Could you check a few things on this model? Use its own coordinates, in mm. Give positions to 0.01 mm unless a question says otherwise; leave off trailing zeros. Loops run counter-clockwise (first coordinate to the right, second up) from the corner with the lowest first, then second, coordinate; pieces in that order, holes last. Notation, with made-up numbers: M -4,71 L 49,71 A35 cw 49,104 Z; hole C 75,68 d9. An arc over 180 degrees is marked long. Answer in a Markdown table with one row per item. Add a question column.
1. If we section it at B-B on x = -17.5: List the corners of the cut face in (y, z) for me, then the cut area to 3 significant figures.
2. If we section it at D-D on y = 4: Count the separate pieces of the cut face and the enclosed holes in it, then the cut area to 3 significant figures.
3. I'm going to push flat-ended pins straight in: pin 1 Ø5 at (x, z) = (24.89, 60.6) entering from +Y; pin 2 Ø1.6 at (x, y) = (24, 3.5) entering from +Z; pin 3 Ø2.5 at (x, y) = (26, 3.5) entering from -Z. Where does each tip first touch, or does it pass through?
4. If we section it at A-A on z = 71: List the corners of the cut face in (x, y) for me.
5. If we section it at C-C on z = 9.22: List the corners of the cut face in (x, y) for me, then the cut area to 3 significant figures.
6. I need wall thicknesses on line 1 along X through (y, z) = (0.65, 83); line 2 along Z through (x, y) = (26, 2.75); line 3 along Z through (x, y) = (-25.5, 1.75). Which ranges of each line are inside material? Lowest first, please. Write a range as from..to.
```python
from build123d import *

# Parameters (mm, degrees)
SKETCH1_R           = 1.5
SKETCH1_R_2         = 6.5
SKETCH1_R_3         = 5.5
BOSS_EXTRUDE1_DEPTH = 6
FILLET1_R           = 10
SKETCH2_R           = 4
CUT_EXTRUDE1_DEPTH  = 3
SKETCH1_3_R         = 5.5
SKETCH1_3_R_2       = 3.5
BOSS_EXTRUDE2_DEPTH = 3
SKETCH3_W           = 3.3
SKETCH3_H           = 7.5
SKETCH3_H_2         = 1
SKETCH3_W_2         = 1.15
SKETCH3_H_3         = 4.1
SKETCH3_H_4         = 2.4
CUT_EXTRUDE2_DEPTH  = 10


with BuildPart() as part:
    # Sketch1 → Boss-Extrude1 (new body)
    with BuildSketch(Plane(origin=(0, 0, 0), x_dir=(1, 0, 0), z_dir=(0, 1, 0))):
        Polygon((17.441626812, 0.78), (-17.441626812, 0.78), (-35, -35.22), (-35, -94.22), (-12.5, -94.22), (-12.5, -88.22), (12.5, -88.22), (12.5, -94.22), (35, -94.22), (35, -35.22), align=None)
        with Locations(Location((-24.889613301, -70.60075616, 0), (0, 0, 270))):
            Circle(SKETCH1_R, mode=Mode.SUBTRACT)
        with Locations(Location((-24.889613301, -60.60075616, 0), (0, 0, 270))):
            Circle(SKETCH1_R, mode=Mode.SUBTRACT)
        with Locations(Location((24.889613301, -70.60075616, 0), (0, 0, 270))):
            Circle(SKETCH1_R, mode=Mode.SUBTRACT)
        with Locations(Location((10.3, -65.60075616, 0), (0, 0, 270))):
            Circle(SKETCH1_R_2, mode=Mode.SUBTRACT)
        with Locations(Location((24.889613301, -60.60075616, 0), (0, 0, 270))):
            Circle(SKETCH1_R, mode=Mode.SUBTRACT)
        with Locations(Location((-17.5, -33.65200814, 0), (0, 0, 270))):
            Circle(SKETCH1_R_3, mode=Mode.SUBTRACT)
        with Locations(Location((-8.607476274, -9.22, 0), (0, 0, 270))):
            Circle(SKETCH1_R_3, mode=Mode.SUBTRACT)
        with Locations(Location((17.5, -33.65200814, 0), (0, 0, 270))):
            Circle(SKETCH1_R_3, mode=Mode.SUBTRACT)
        with Locations(Location((8.607476274, -9.22, 0), (0, 0, 270))):
            Circle(SKETCH1_R_3, mode=Mode.SUBTRACT)
    extrude(amount=BOSS_EXTRUDE1_DEPTH)

    # Fillet1
    fillet1_edges = [part.edges().sort_by_distance(p)[0] for p in [
        (-35, 3, 35.22),
        (-17.441626812, 3, -0.78),
        (17.441626812, 3, -0.78),
        (35, 3, 35.22),
    ]]
    fillet(fillet1_edges, radius=FILLET1_R)

    # Sketch2 → Cut-Extrude1 (cut)
    with BuildSketch(Plane(origin=(0, 6, 0), x_dir=(1, 0, 0), z_dir=(0, 1, 0))):
        with Locations(Location((24.889613301, -60.60075616, 0), (0, 0, 270))):
            Circle(SKETCH2_R)
        with Locations(Location((24.889613301, -70.60075616, 0), (0, 0, 270))):
            Circle(SKETCH2_R)
        with Locations(Location((-24.889613301, -60.60075616, 0), (0, 0, 270))):
            Circle(SKETCH2_R)
        with Locations(Location((-24.889613301, -70.60075616, 0), (0, 0, 270))):
            Circle(SKETCH2_R)
    extrude(amount=-CUT_EXTRUDE1_DEPTH, mode=Mode.SUBTRACT)

    # Sketch1_3 → Boss-Extrude2 (add)
    # profile 1 of 4: a face of its own
    with BuildSketch(Plane(origin=(0, 0, 0), x_dir=(1, 0, 0), z_dir=(0, 1, 0))):
        with Locations(Location((-17.5, -33.65200814, 0), (0, 0, 270))):
            Circle(SKETCH1_3_R)
        with Locations(Location((-17.5, -33.65200814, 0), (0, 0, 270))):
            Circle(SKETCH1_3_R_2, mode=Mode.SUBTRACT)
    # profile 2 of 4: a face of its own
    with BuildSketch(Plane(origin=(0, 0, 0), x_dir=(1, 0, 0), z_dir=(0, 1, 0))):
        with Locations(Location((-8.607476274, -9.22, 0), (0, 0, 270))):
            Circle(SKETCH1_3_R)
        with Locations(Location((-8.607476274, -9.22, 0), (0, 0, 270))):
            Circle(SKETCH1_3_R_2, mode=Mode.SUBTRACT)
    # profile 3 of 4: a face of its own
    with BuildSketch(Plane(origin=(0, 0, 0), x_dir=(1, 0, 0), z_dir=(0, 1, 0))):
        with Locations(Location((17.5, -33.65200814, 0), (0, 0, 270))):
            Circle(SKETCH1_3_R)
        with Locations(Location((17.5, -33.65200814, 0), (0, 0, 270))):
            Circle(SKETCH1_3_R_2, mode=Mode.SUBTRACT)
    # profile 4 of 4: a face of its own
    with BuildSketch(Plane(origin=(0, 0, 0), x_dir=(1, 0, 0), z_dir=(0, 1, 0))):
        with Locations(Location((8.607476274, -9.22, 0), (0, 0, 270))):
            Circle(SKETCH1_3_R)
        with Locations(Location((8.607476274, -9.22, 0), (0, 0, 270))):
            Circle(SKETCH1_3_R_2, mode=Mode.SUBTRACT)
    extrude(amount=BOSS_EXTRUDE2_DEPTH)

    # Sketch3 → Cut-Extrude2 (cut)
    with BuildSketch(Plane(origin=(0, 6, 0), x_dir=(1, 0, 0), z_dir=(0, 1, 0))):
        with Locations((23.75, -90.47)):
            Rectangle(SKETCH3_W, SKETCH3_H)
        Polygon((26.55, -85.72), (25.4, -85.72), (25.4, -86.72), (27.75, -86.72), (27.75, -85.72), align=None)
        with Locations((23.75, -86.22)):
            Rectangle(SKETCH3_W, SKETCH3_H_2)
        Polygon((22.1, -85.72), (20.95, -85.72), (19.75, -85.72), (19.75, -86.72), (22.1, -86.72), align=None)
        with Locations((21.525, -83.67)):
            Rectangle(SKETCH3_W_2, SKETCH3_H_3)
        with Locations((23.75, -83.67)):
            Rectangle(SKETCH3_W, SKETCH3_H_3)
        with Locations((25.975, -83.67)):
            Rectangle(SKETCH3_W_2, SKETCH3_H_3)
        with Locations((23.75, -80.42)):
            Rectangle(SKETCH3_W, SKETCH3_H_4)
    cut_extrude2 = extrude(amount=-CUT_EXTRUDE2_DEPTH, mode=Mode.SUBTRACT)

    # Mirror1: Cut-Extrude2 across plane
    add(cut_extrude2.mirror(Plane(origin=(0, 0, 0), x_dir=(0, 0, 1), z_dir=(1, 0, 0))), mode=Mode.SUBTRACT)


solid = part.part
```
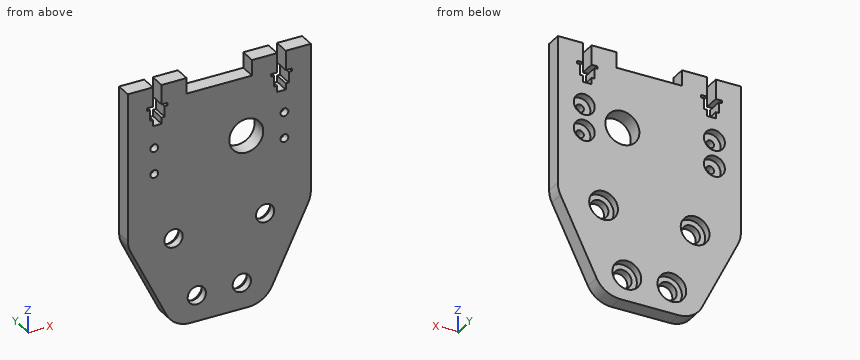
Results:
| question | item | result |
|---|---|---|
| 1 | outline | M 0,1.46 L 6,1.46 L 6,28.15 L 3,28.15 L 3,30.15 L 0,30.15 Z; M 0,37.15 L 3,37.15 L 3,39.15 L 6,39.15 L 6,94.22 L 0,94.22 Z |
| 1 | area | 503 mm2 |
| 2 | separate pieces | 1 |
| 2 | enclosed holes | 9 |
| 2 | area | 5,010 mm2 |
| 3 | pin 1 | y = 3 |
| 3 | pin 2 | z = 79.22 |
| 3 | pin 3 | z = 14.2 |
| 4 | outline | M -35,0 L -26.34,0 L -26.34,3 L -28.87,3 L -28.87,6 L -35,6 Z; M -23.44,0 L 6.68,0 L 6.68,6 L -20.91,6 L -20.91,3 L -23.44,3 Z; M 13.92,0 L 23.44,0 L 23.44,3 L 20.91,3 L 20.91,6 L 13.92,6 Z; M 26.34,0 L 35,0 L 35,6 L 28.87,6 L 28.87,3 L 26.34,3 Z |
| 5 | outline | M -22.32,0 L -12.11,0 L -12.11,3 L -14.11,3 L -14.11,6 L -22.32,6 Z; M -5.11,0 L 5.11,0 L 5.11,3 L 3.11,3 L 3.11,6 L -3.11,6 L -3.11,3 L -5.11,3 Z; M 12.11,0 L 22.32,0 L 22.32,6 L 14.11,6 L 14.11,3 L 12.11,3 Z |
| 5 | area | 160 mm2 |
| 6 | line 1 | -35..-26.55, -20.95..20.95, 26.55..35 |
| 6 | line 2 | 16.77..59.59, 61.61..69.59, 71.61..81.62, 86.72..94.22 |
| 6 | line 3 | 15.74..59.23, 61.97..69.23, 71.97..81.62, 86.72..94.22 |
